Geometry check sheet. Reference: drawing and pictorial views, mm from the part's lowest x, y, z. Coordinates: 2 decimals unless noted, no trailing zeros. Write each loop counter-clockwise with the first axis right and the second up, starting at its lowest first coordinate (ties: lowest second). Pieces come first, ordered by that corner, then holes. Notation, with made-up numbers: (65.25, 5.25) -> (92.25, 5.25) arc R20 cw to (92.25, 30.25) -> close; hole circle Ø7 at (3.25, 7.25). An arc over 180 degrees is marked (long way). Use a Markdown table: item, result. Add a question column.
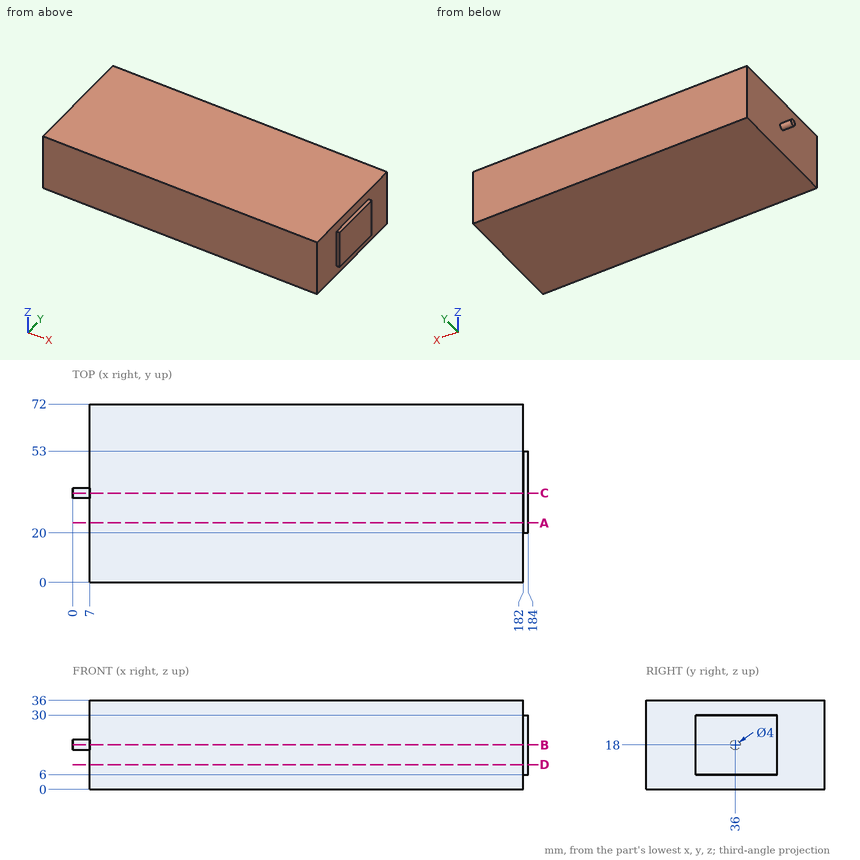
1) Thickness scan on L1, parallel to X at y = 23, z = 18; L2, parallel to X at y = 18, z = 34.5. Record the ranges inside material, lowest first.
2) Gauge pin test, flat ends, axial feed: pin 1 (12 mm diameter, centred on x = 21, y = 24, fed in from -Z); pin 2 (1.5 mm diameter, centred on y = 63.5, z = 8, fed in from +X); pin 3 (0.6 mm diameter, centred on x = 183, z = 23.5, fed in from +Y); pin 4 (1 mm diameter, centred on x = 183, y = 37.5, fed in from -Z). Record the tip position at first contact, or that the pin passes through.
3) Cross-section at C-C on y = 36. Record the boundary of the cut face in (x, z).
4) Cross-section at D-D on z = 10. Record the boundary of the cut face in (x, y), then the cut area to 3 significant figures.
5) Cross-section at A-A on y = 24. Record the boundary of the cut face in (x, z).
6) Cross-section at B-B on z = 18. Record the boundary of the cut face in (x, y), then the cut area to 3 significant figures.
Returned:
| question | item | result |
|---|---|---|
| 1 | L1 | x = 7 to 184 |
| 1 | L2 | x = 7 to 182 |
| 2 | pin 1 | stops at z = 0 |
| 2 | pin 2 | stops at x = 182 |
| 2 | pin 3 | stops at y = 53 |
| 2 | pin 4 | stops at z = 6 |
| 3 | outline | (0, 16) -> (7, 16) -> (7, 0) -> (182, 0) -> (182, 6) -> (184, 6) -> (184, 30) -> (182, 30) -> (182, 36) -> (7, 36) -> (7, 20) -> (0, 20) -> close |
| 4 | outline | (7, 0) -> (182, 0) -> (182, 20) -> (184, 20) -> (184, 53) -> (182, 53) -> (182, 72) -> (7, 72) -> close |
| 4 | area | 12,700 mm² |
| 5 | outline | (7, 0) -> (182, 0) -> (182, 6) -> (184, 6) -> (184, 30) -> (182, 30) -> (182, 36) -> (7, 36) -> close |
| 6 | outline | (0, 34) -> (7, 34) -> (7, 0) -> (182, 0) -> (182, 20) -> (184, 20) -> (184, 53) -> (182, 53) -> (182, 72) -> (7, 72) -> (7, 38) -> (0, 38) -> close |
| 6 | area | 12,700 mm² |
